Build history of the part. All positions in model axes, mm. Face numbers are marked on the shaded views. A direction names the side the tool comes from. Round coordinates to 2 decimals unless told otherwise and drop trailing zeros. Write each loop counter-clockwise with the first axis right and the second up, starting at its lowest first coordinate (ties: lowest second). Pieces come first, ordered by that corner, then holes. Notation, with made-up numbers: (44, -38.75) - (59, -38.75) arc R24 ccw to (59, -26.75) - close; hole circle Ø10 at (55.5, 25). An arc over 180 degrees is marked (long way). Answer as a JSON object with one key per item and string values. Group by question number.
Item 1: Slice it at A-A, the plane x = 6.5. List the corners of the cut face in (y, z).
Item 2: Which spindle directions (+Z, -Z, +X, -X, +Y, -Y) get a long thin tool onto all of the face, cutting with end or side? Do the marked faces 4, 5 and 6. Say none if no direction does.
Item 3: Flat gauge pins, fed straight in: pin 1 (3 mm diameter, centred on y = 0.5, z = 10, fed in from -X); pin 2 (1 mm diameter, centred on y = -7, z = 13, fed in from +X); pin 3 (7.5 mm diameter, centred on x = 6.5, z = 4.5, fed in from +Y); pin 4 (8 mm diameter, centred on x = 30, y = 5, fed in from -Z). Where does each tip first touch, or does it go through?
Item 4: Slice it at C-C, the plane y = 2. List the corners of the cut face in (x, z).
Item 5: Two-plate mould, pull along Z, no slides. Class the marked faces 1, 2 and 3: +Z half, -Z half, draft (parallel to the pull), parting line (faces both ways), or undercut.
Item 6: Slice it at B-B, the plane z = 11. List the corners of the cut face in (x, y), then the cut area to 3 significant figures.
Item 7: Slice it at D-D, the plane z = 18. List the corners of the cut face in (x, y).
Item 8: Probe line 1 (Z direction, x = -9.5, y = 6.5); line 2 (Z direction, x = -7.5, y = 2.75); line 3 (X direction, y = 1.25, z = 22.5). List the from-to ranges inside material, lowest first. Write a range as from..to.
from build123d import *

# Parameters (mm, degrees)
ESQUISSE1_W             = 101
ESQUISSE1_H             = 19
BOSS_EXTRU_1_DEPTH      = 15
ESQUISSE2_W             = 119
ESQUISSE2_H             = 22
BOSS_EXTRU_2_DEPTH      = 1.8
ESQUISSE3_W             = 16
ESQUISSE3_H             = 8
ENL_V_MAT_EXTRU_1_DEPTH = 66.136318594
ESQUISSE4_W             = 8
ESQUISSE4_H             = 1
ESQUISSE4_H_2           = 13
ENL_V_MAT_EXTRU_2_DEPTH = 97.120965455
ESQUISSE5_W             = 28
ESQUISSE5_H             = 10
BOSS_EXTRU_3_DEPTH      = 6
ESQUISSE7_W             = 2.54
ESQUISSE7_H             = 12.7
BOSS_EXTRU_4_DEPTH      = 10


with BuildPart() as part:
    # Esquisse1 → Boss.-Extru.1 (new body)
    with BuildSketch(Plane.XY):
        Rectangle(ESQUISSE1_W, ESQUISSE1_H)
    extrude(amount=BOSS_EXTRU_1_DEPTH)

    # Esquisse2 → Boss.-Extru.2 (add)
    with BuildSketch(Plane.XY.offset(15)):
        Rectangle(ESQUISSE2_W, ESQUISSE2_H)
    extrude(amount=BOSS_EXTRU_2_DEPTH)

    # Esquisse3 → Enlèv. mat.-Extru.1 (cut, through all)
    with BuildSketch(Plane(origin=(0, 9.5, 0), x_dir=(1, 0, 0), z_dir=(0, 1, 0))):
        with Locations((-8, -11)):
            Rectangle(ESQUISSE3_W, ESQUISSE3_H)
        with Locations((8, -11)):
            Rectangle(ESQUISSE3_W, ESQUISSE3_H)
        with Locations((42.5, -11)):
            Rectangle(ESQUISSE3_W, ESQUISSE3_H)
        with Locations((-42.5, -11)):
            Rectangle(ESQUISSE3_W, ESQUISSE3_H)
    extrude(amount=-ENL_V_MAT_EXTRU_1_DEPTH, mode=Mode.SUBTRACT)

    # Esquisse4 → Enlèv. mat.-Extru.2 (cut, through all)
    with BuildSketch(Plane.ZY.offset(34.5)):
        with Locations((11, 9)):
            Rectangle(ESQUISSE4_W, ESQUISSE4_H)
        with Locations((11, 0)):
            Rectangle(ESQUISSE4_W, ESQUISSE4_H_2)
        with Locations((11, -9)):
            Rectangle(ESQUISSE4_W, ESQUISSE4_H)
    extrude(amount=-ENL_V_MAT_EXTRU_2_DEPTH, mode=Mode.SUBTRACT)

    # Esquisse5 → Boss.-Extru.3 (add)
    with BuildSketch(Plane(origin=(0, 0, 15), x_dir=(-1, 0, 0), z_dir=(0, 0, -1))):
        Rectangle(ESQUISSE5_W, ESQUISSE5_H)
    extrude(amount=BOSS_EXTRU_3_DEPTH)

    # Esquisse7 → Boss.-Extru.4 (add)
    with BuildSketch(Plane(origin=(0, 0, 15), x_dir=(-1, 0, 0), z_dir=(0, 0, -1))):
        with Locations((-53.48, 0)):
            Rectangle(ESQUISSE7_W, ESQUISSE7_H)
        with Locations((53.48, 0)):
            Rectangle(ESQUISSE7_W, ESQUISSE7_H)
    extrude(amount=-BOSS_EXTRU_4_DEPTH)


solid = part.part
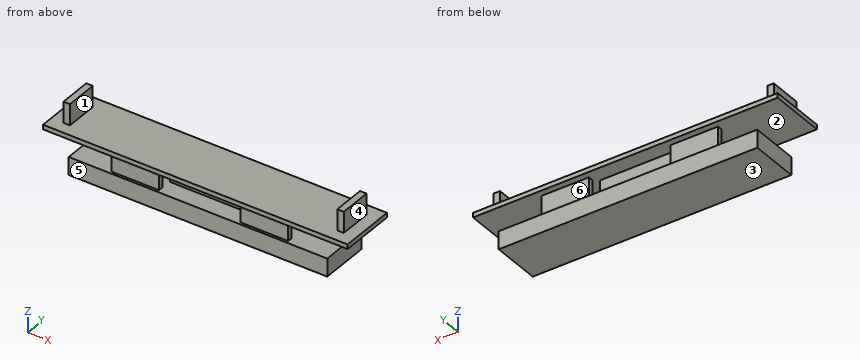
Geometry says:
{
 "1": {"outline": "(-11, 15) - (-5, 15) - (-5, 9) - (5, 9) - (5, 15) - (11, 15) - (11, 16.8) - (-11, 16.8) - close; (-9.5, 0) - (9.5, 0) - (9.5, 7) - (-9.5, 7) - close"},
 "2": {"face 4": "+Z, +X, +Y, -Y", "face 5": "-Z, +X, -X, -Y", "face 6": "+X, -X, +Y"},
 "3": {"pin 1": "stops at x = -14", "pin 2": "stops at x = 34.5", "pin 3": "stops at y = 9.5", "pin 4": "stops at z = 0"},
 "4": {"outline": "(-59.5, 15) - (-14, 15) - (-14, 9) - (14, 9) - (14, 15) - (59.5, 15) - (59.5, 16.8) - (54.75, 16.8) - (54.75, 25) - (52.21, 25) - (52.21, 16.8) - (-52.21, 16.8) - (-52.21, 25) - (-54.75, 25) - (-54.75, 16.8) - (-59.5, 16.8) - close; (-50.5, 0) - (50.5, 0) - (50.5, 7) - (-50.5, 7) - close"},
 "5": {"face 1": "draft", "face 2": "undercut", "face 3": "-Z half"},
 "6": {"outline": "(-34.5, -8.5) - (-16, -8.5) - (-16, -6.5) - (-34.5, -6.5) - close; (-34.5, 6.5) - (-16, 6.5) - (-16, 8.5) - (-34.5, 8.5) - close; (-14, -5) - (14, -5) - (14, 5) - (-14, 5) - close; (16, -8.5) - (34.5, -8.5) - (34.5, -6.5) - (16, -6.5) - close; (16, 6.5) - (34.5, 6.5) - (34.5, 8.5) - (16, 8.5) - close", "area": "428 mm^2"},
 "7": {"outline": "(-54.75, -6.35) - (-52.21, -6.35) - (-52.21, 6.35) - (-54.75, 6.35) - close; (52.21, -6.35) - (54.75, -6.35) - (54.75, 6.35) - (52.21, 6.35) - close"},
 "8": {"line 1": "z = 0..7, 15..16.8", "line 2": "z = 0..7, 9..16.8", "line 3": "x = -54.75..-52.21, 52.21..54.75"}
}
